Design review of the part built by this model. Coordinates are the model's own, in mm. Coordinates: 2 decimals unless noted, no trailing zeros. Order: outer loops, then holes, each group sorted by start corner. A loop starts at its lowest first (then second) coordinate and runs counter-clockwise, first axis right, second up. Notation, with made-up numbers: M 85.25,22 L 89.25,22 A13 cw 89.25,40 Z; hole C 3,-16.75 d7. An arc over 180 degrees is marked long. Answer as a JSON object with one key per item and string values.
from build123d import *

# Parameters (mm, degrees)
F1_DEPTH = 5.08


with BuildPart() as f1:
    # F0 (on Front) → F1 (new body)
    with BuildSketch(Plane.XZ):
        with BuildLine():
            Line((-30.099, -178.2621852636), (-42.799, -178.2621852636))
            ThreePointArc((-42.799, -178.2621852636), (-30.263463128, -208.5256483916), (0, -221.0611852636))
            Line((0, -221.0611852636), (0, -208.3611852636))
            ThreePointArc((0, -208.3611852636), (-21.2832070069, -199.5453922706), (-30.099, -178.2621852636))
        make_face()
        with BuildLine():
            ThreePointArc((0, -221.0611852636), (30.263463128, -208.5256483916), (42.799, -178.2621852636))
            Line((42.799, -178.2621852636), (30.099, -178.2621852636))
            ThreePointArc((30.099, -178.2621852636), (21.2832070069, -199.5453922706), (0, -208.3611852636))
            Line((0, -208.3611852636), (0, -221.0611852636))
        make_face()
        with BuildLine():
            Line((42.799, 164.6378147364), (30.099, 164.6378147364))
            Line((30.099, 164.6378147364), (30.099, 134.2107774176))
            ThreePointArc((30.099, 134.2107774176), (39.4965916378, 148.1522559045), (42.799, 164.6378147364))
        make_face()
        with BuildLine():
            ThreePointArc((42.799, -178.2621852636), (39.4965916378, -161.7766264317), (30.099, -147.8351479448))
            Line((30.099, -147.8351479448), (30.099, -178.2621852636))
            Line((30.099, -178.2621852636), (42.799, -178.2621852636))
        make_face()
        with BuildLine():
            Line((-30.099, 134.2107774176), (-30.099, 164.6378147364))
            Line((-30.099, 164.6378147364), (-42.799, 164.6378147364))
            ThreePointArc((-42.799, 164.6378147364), (-39.4965916378, 148.1522559045), (-30.099, 134.2107774176))
        make_face()
        with BuildLine():
            Line((-30.099, -178.2621852636), (-30.099, -147.8351479448))
            ThreePointArc((-30.099, -147.8351479448), (-39.4965916378, -161.7766264317), (-42.799, -178.2621852636))
            Line((-42.799, -178.2621852636), (-30.099, -178.2621852636))
        make_face()
        with BuildLine():
            ThreePointArc((15.0495, -138.1964024715), (7.6478416327, -136.1520330511), (0, -135.4631852636))
            Line((0, -135.4631852636), (0, -148.1631852636))
            ThreePointArc((0, -148.1631852636), (7.7901944385, -149.1887838182), (15.0495, -152.1956866351))
            Line((15.0495, -152.1956866351), (15.0495, -138.1964024715))
        make_face()
        with BuildLine():
            Line((0, -148.1631852636), (0, -135.4631852636))
            ThreePointArc((0, -135.4631852636), (-7.6478416327, -136.1520330511), (-15.0495, -138.1964024715))
            Line((-15.0495, -138.1964024715), (-15.0495, -152.1956866351))
            ThreePointArc((-15.0495, -152.1956866351), (-7.7901944385, -149.1887838182), (0, -148.1631852636))
        make_face()
        with BuildLine():
            Line((0, 121.8388147364), (0, 134.5388147364))
            ThreePointArc((0, 134.5388147364), (-7.7901944385, 135.5644132909), (-15.0495, 138.5713161079))
            Line((-15.0495, 138.5713161079), (-15.0495, 124.5720319442))
            ThreePointArc((-15.0495, 124.5720319442), (-7.6478416327, 122.5276625239), (0, 121.8388147364))
        make_face()
        with BuildLine():
            ThreePointArc((15.0495, 138.5713161079), (7.7901944385, 135.5644132909), (0, 134.5388147364))
            Line((0, 134.5388147364), (0, 121.8388147364))
            ThreePointArc((0, 121.8388147364), (7.6478416327, 122.5276625239), (15.0495, 124.5720319442))
            Line((15.0495, 124.5720319442), (15.0495, 138.5713161079))
        make_face()
        with BuildLine():
            ThreePointArc((30.099, 164.6378147364), (26.0664986285, 149.5883147364), (15.0495, 138.5713161079))
            Line((15.0495, 138.5713161079), (15.0495, 124.5720319442))
            ThreePointArc((15.0495, 124.5720319442), (23.0829616089, 128.5971254483), (30.099, 134.2107774176))
            Line((30.099, 134.2107774176), (30.099, 164.6378147364))
        make_face()
        with BuildLine():
            ThreePointArc((30.099, -147.8351479448), (23.0829616089, -142.2214959755), (15.0495, -138.1964024715))
            Line((15.0495, -138.1964024715), (15.0495, -152.1956866351))
            ThreePointArc((15.0495, -152.1956866351), (26.0664986285, -163.2126852636), (30.099, -178.2621852636))
            Line((30.099, -178.2621852636), (30.099, -147.8351479448))
        make_face()
        with BuildLine():
            Line((-15.0495, -152.1956866351), (-15.0495, -138.1964024715))
            ThreePointArc((-15.0495, -138.1964024715), (-23.0829616089, -142.2214959755), (-30.099, -147.8351479448))
            Line((-30.099, -147.8351479448), (-30.099, -178.2621852636))
            ThreePointArc((-30.099, -178.2621852636), (-26.0664986285, -163.2126852636), (-15.0495, -152.1956866351))
        make_face()
        with BuildLine():
            Line((-15.0495, 124.5720319442), (-15.0495, 138.5713161079))
            ThreePointArc((-15.0495, 138.5713161079), (-26.0664986285, 149.5883147364), (-30.099, 164.6378147364))
            Line((-30.099, 164.6378147364), (-30.099, 134.2107774176))
            ThreePointArc((-30.099, 134.2107774176), (-23.0829616089, 128.5971254483), (-15.0495, 124.5720319442))
        make_face()
        with BuildLine():
            Line((-42.799, 164.6378147364), (-30.099, 164.6378147364))
            ThreePointArc((-30.099, 164.6378147364), (-21.2832070069, 185.9210217433), (0, 194.7368147364))
            Line((0, 194.7368147364), (0, 207.4368147364))
            ThreePointArc((0, 207.4368147364), (-30.263463128, 194.9012778644), (-42.799, 164.6378147364))
        make_face()
        with BuildLine():
            ThreePointArc((0, 194.7368147364), (21.2832070069, 185.9210217433), (30.099, 164.6378147364))
            Line((30.099, 164.6378147364), (42.799, 164.6378147364))
            ThreePointArc((42.799, 164.6378147364), (30.263463128, 194.9012778644), (0, 207.4368147364))
            Line((0, 207.4368147364), (0, 194.7368147364))
        make_face()
        with BuildLine():
            ThreePointArc((42.799, 164.6378147364), (39.4965916378, 148.1522559045), (30.099, 134.2107774176))
            Line((30.099, 134.2107774176), (30.099, -147.8351479448))
            ThreePointArc((30.099, -147.8351479448), (39.4965916378, -161.7766264317), (42.799, -178.2621852636))
            Line((42.799, -178.2621852636), (42.799, 164.6378147364))
        make_face()
        with BuildLine():
            Line((-30.099, -147.8351479448), (-30.099, 134.2107774176))
            ThreePointArc((-30.099, 134.2107774176), (-39.4965916378, 148.1522559045), (-42.799, 164.6378147364))
            Line((-42.799, 164.6378147364), (-42.799, -178.2621852636))
            ThreePointArc((-42.799, -178.2621852636), (-39.4965916378, -161.7766264317), (-30.099, -147.8351479448))
        make_face()
        with BuildLine():
            Line((0, -135.4631852636), (0, 121.8388147364))
            ThreePointArc((0, 121.8388147364), (-7.6478416327, 122.5276625239), (-15.0495, 124.5720319442))
            Line((-15.0495, 124.5720319442), (-15.0495, -138.1964024715))
            ThreePointArc((-15.0495, -138.1964024715), (-7.6478416327, -136.1520330511), (0, -135.4631852636))
        make_face()
        with BuildLine():
            ThreePointArc((15.0495, 124.5720319442), (7.6478416327, 122.5276625239), (0, 121.8388147364))
            Line((0, 121.8388147364), (0, -135.4631852636))
            ThreePointArc((0, -135.4631852636), (7.6478416327, -136.1520330511), (15.0495, -138.1964024715))
            Line((15.0495, -138.1964024715), (15.0495, 124.5720319442))
        make_face()
        with BuildLine():
            ThreePointArc((30.099, 134.2107774176), (23.0829616089, 128.5971254483), (15.0495, 124.5720319442))
            Line((15.0495, 124.5720319442), (15.0495, -138.1964024715))
            ThreePointArc((15.0495, -138.1964024715), (23.0829616089, -142.2214959755), (30.099, -147.8351479448))
            Line((30.099, -147.8351479448), (30.099, 134.2107774176))
        make_face()
        with BuildLine():
            Line((-15.0495, -138.1964024715), (-15.0495, 124.5720319442))
            ThreePointArc((-15.0495, 124.5720319442), (-23.0829616089, 128.5971254483), (-30.099, 134.2107774176))
            Line((-30.099, 134.2107774176), (-30.099, -147.8351479448))
            ThreePointArc((-30.099, -147.8351479448), (-23.0829616089, -142.2214959755), (-15.0495, -138.1964024715))
        make_face()
    extrude(amount=F1_DEPTH)


solid = f1.part
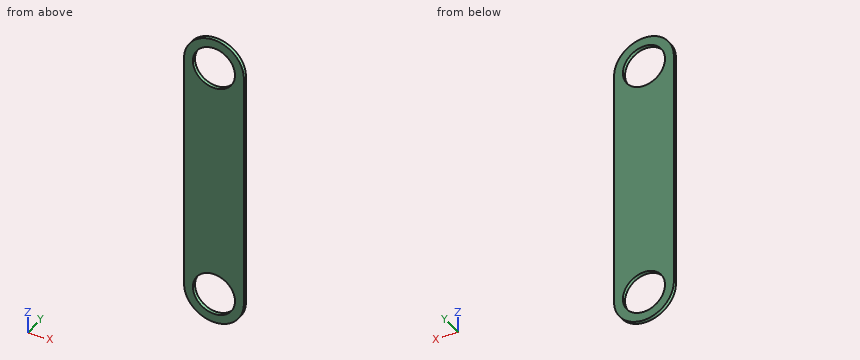
1) To check wall thickness, follow L1, parallel to Z at x = 17.5, y = -4.9; L2, parallel to Z at x = -17, y = -0.5; L3, parallel to X at y = -1, z = -178. State the ranges of each line that lie inside material, in increasing order.
Taken from the geometry:
{"L1": "z = -217.32 to -202.75, -153.77 to 140.15, 189.13 to 203.7", "L2": "z = -217.54 to -203.1, -153.42 to 139.8, 189.48 to 203.92", "L3": "x = -42.8 to -30.1, 30.1 to 42.8"}
2) Add section C-C (x = -37). State the section outline as (y, z) points, and give its area (3 significant figures).
Taken from the geometry:
{"outline": "M -5.08,-199.77 L 0,-199.77 L 0,186.15 L -5.08,186.15 Z", "area": "1,960 mm2"}
3) Add section B-B (x = 9). State the section outline as (y, z) points, and give its area (3 significant figures).
Taken from the geometry:
{"outline": "M -5.08,-220.1 L 0,-220.1 L 0,-206.98 L -5.08,-206.98 Z; M -5.08,-149.54 L 0,-149.54 L 0,135.92 L -5.08,135.92 Z; M -5.08,193.36 L 0,193.36 L 0,206.48 L -5.08,206.48 Z", "area": "1,580 mm2"}
4) Insertion check: pin 1 Ø2 at (x, y) = (34, -0.5) entering from +Z. The pin has a flat end and moves straight along its axis. Give the tip position at first contact, or say it passes through.
Taken from the geometry:
{"pin 1": "stops at z = 191.89"}
5) Add section A-A (y = -4.1). State the section outline as (x, z) points.
Taken from the geometry:
{"outline": "M -42.8,-178.26 A42.8 ccw 42.8,-178.26 L 42.8,164.64 A42.8 ccw -42.8,164.64 Z; hole C 0,-178.26 d60.2; hole C 0,164.64 d60.2"}
